The listing builds one solid part. Answer for the finished solid, in the listing's coordinates (mm). A direction names the side the tool comes from. Round coordinates to 2 decimals unless told otherwise and drop trailing zeros. Write each loop counter-clockwise with the first axis right and the second up, starting at its lowest first coordinate (ties: lowest second). Pieces come first, ordered by that corner, then holes. Notation, with made-up numbers: (82, 83.5) - (137, 83.5) arc R26 cw to (137, 108.5) - close; hole circle Ø9 at (27.25, 39.5). An arc over 180 degrees is marked (long way). Use a Markdown table: item, result. Add a question column.
1) A cutting plane is placed at A-A (y = -12.25). Give the vertices of the cut face in (x, z), then the cut area to 3 significant figures.
2) Find the intervals of material crossed by probe 1 along X at (y, z) = (-7.75, 0); probe 2 along Y at (x, z) = (5, 7); probe 3 along X at (y, z) = (-4.5, 0), in increasing order. Write a range as from..to.
3) A cutting plane is placed at B-B (x = -2). Give the vertices of the cut face in (y, z), then the cut area to 3 significant figures.
4) A tool of negligible diameter and unlimited length cuts with its end or side. For faces 1 (the cylindrical face through (-10.316, -8.381, -7.91)), 2 (the flat face through (-8, -5, -14.4)), 3 (the flat face through (8.4, -5, 14.1)), 4 (the flat face through (16.3, -5, 0)), 5 (the flat face through (8.4, -5, -14.1)), from which of +Z, -Z, +X, -X, +Y, -Y can it reach the whole face along a straight path? Write none if from no direction.
5) Each of these flat-tipped pins is pushed along its axis until it touches: P1, Ø2, axis at x = -4, z = 11, coming from the +Y side; P2, Ø6, axis at x = 11, y = -6, coming from the +Z side; P3, Ø4, axis at y = -11, z = -6, coming from the +X side. Where does it stop, or does it pass through?
6) A cutting plane is placed at C-C (y = -14.5). Give the vertices of the cut face in (x, z).
```python
from build123d import *

# Parameters (mm, degrees)
F0_R     = 16
F0_R_2   = 13
F1_DEPTH = 5
F2_R     = 13
F3_DEPTH = 13
F4_R     = 7.5
F5_DEPTH = 1
F6_R     = 5


with BuildPart() as f1:
    # F0 (on Front) → F1 (new body)
    with BuildSketch(Plane.XZ):
        Circle(F0_R)
        Circle(F0_R_2, mode=Mode.SUBTRACT)
    extrude(amount=F1_DEPTH)

    # F2 (on face) → F3 (join)
    with BuildSketch(Plane.XZ.offset(5)):
        with BuildLine():
            Line((6.3508529611, 16), (-6.3508529611, 16))
            ThreePointArc((-6.3508529611, 16), (-8.8508529611, 15.3301270189), (-10.68097998, 13.5))
            Line((-10.68097998, 13.5), (-17.0318329411, 2.5))
            ThreePointArc((-17.0318329411, 2.5), (-17.7017059222, 0), (-17.0318329411, -2.5))
            Line((-17.0318329411, -2.5), (-10.68097998, -13.5))
            ThreePointArc((-10.68097998, -13.5), (-8.8508529611, -15.3301270189), (-6.3508529611, -16))
            Line((-6.3508529611, -16), (6.3508529611, -16))
            ThreePointArc((6.3508529611, -16), (8.8508529611, -15.3301270189), (10.68097998, -13.5))
            Line((10.68097998, -13.5), (17.0318329411, -2.5))
            ThreePointArc((17.0318329411, -2.5), (17.7017059222, 0), (17.0318329411, 2.5))
            Line((17.0318329411, 2.5), (10.68097998, 13.5))
            ThreePointArc((10.68097998, 13.5), (8.8508529611, 15.3301270189), (6.3508529611, 16))
        make_face()
        Circle(F2_R, mode=Mode.SUBTRACT)
    extrude(amount=F3_DEPTH)

    # F4 (on face) → F5 (join)
    with BuildSketch(Plane.XZ.offset(18)):
        with BuildLine():
            Line((6.3508529611, 16), (-6.3508529611, 16))
            ThreePointArc((-6.3508529611, 16), (-8.8508529611, 15.3301270189), (-10.68097998, 13.5))
            Line((-10.68097998, 13.5), (-17.0318329411, 2.5))
            ThreePointArc((-17.0318329411, 2.5), (-17.7017059222, 0), (-17.0318329411, -2.5))
            Line((-17.0318329411, -2.5), (-10.68097998, -13.5))
            ThreePointArc((-10.68097998, -13.5), (-8.8508529611, -15.3301270189), (-6.3508529611, -16))
            Line((-6.3508529611, -16), (6.3508529611, -16))
            ThreePointArc((6.3508529611, -16), (8.8508529611, -15.3301270189), (10.68097998, -13.5))
            Line((10.68097998, -13.5), (17.0318329411, -2.5))
            ThreePointArc((17.0318329411, -2.5), (17.7017059222, 0), (17.0318329411, 2.5))
            Line((17.0318329411, 2.5), (10.68097998, 13.5))
            ThreePointArc((10.68097998, 13.5), (8.8508529611, 15.3301270189), (6.3508529611, 16))
        make_face()
        Circle(F4_R, mode=Mode.SUBTRACT)
    extrude(amount=-F5_DEPTH)

    # F6
    f6_edges = [f1.edges().sort_by_distance(p)[0] for p in [
        (13.856406, -18, 8),
    ]]
    fillet(f6_edges, radius=F6_R)


solid = f1.part
```
Entries:
| question | item | result |
|---|---|---|
| 1 | outline | (-17.03, -2.5) - (-10.68, -13.5) arc R5 ccw to (-6.35, -16) - (6.35, -16) arc R5 ccw to (10.68, -13.5) - (17.03, -2.5) arc R5 ccw to (17.03, 2.5) - (10.68, 13.5) arc R5 ccw to (6.35, 16) - (-6.35, 16) arc R5 ccw to (-10.68, 13.5) - (-17.03, 2.5) arc R5 ccw to start; hole circle Ø26 at (0, 0) |
| 1 | area | 348 mm² |
| 2 | probe 1 | x = -17.7..-13, 13..17.7 |
| 2 | probe 2 | y = -18..-17 |
| 2 | probe 3 | x = -16..-13, 13..16 |
| 3 | outline | (-18, -11) arc R5 ccw to (-13, -16) - (-5, -16) - (-5, -15.87) - (0, -15.87) - (0, -12.85) - (-17, -12.85) - (-17, -7.23) - (-18, -7.23) - close; (-18, 7.23) - (-17, 7.23) - (-17, 12.85) - (0, 12.85) - (0, 15.87) - (-5, 15.87) - (-5, 16) - (-13, 16) arc R5 ccw to (-18, 11) - close |
| 3 | area | 113 mm² |
| 4 | face 1 | +Y |
| 4 | face 2 | -Z, -X, +Y |
| 4 | face 3 | +Z, +X, +Y |
| 4 | face 4 | +X, +Y |
| 4 | face 5 | -Z, +X, +Y |
| 5 | P1 | stops at y = -17 |
| 5 | P2 | stops at z = 15.72 |
| 5 | P3 | stops at x = 16.17 |
| 6 | outline | (-16.83, -2.38) - (-10.48, -13.38) arc R4.77 ccw to (-6.35, -15.77) - (6.35, -15.77) arc R4.77 ccw to (10.48, -13.38) - (16.83, -2.38) arc R4.77 ccw to (16.83, 2.38) - (10.48, 13.38) arc R4.77 ccw to (6.35, 15.77) - (-6.35, 15.77) arc R4.77 ccw to (-10.48, 13.38) - (-16.83, 2.38) arc R4.77 ccw to start; hole circle Ø26 at (0, 0) |
